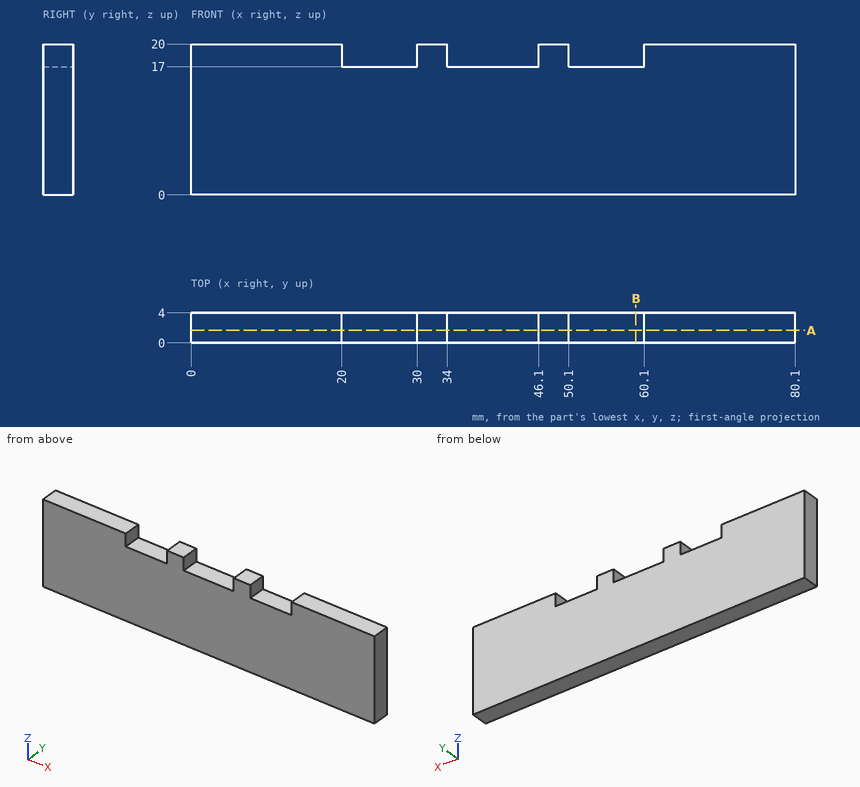
Study the drawing (mm; zero at the part's minimum x, y, z) and answer. Coordinates: 2 decimals unless noted, no trailing zeros. Order: outer loops, then holes, each group sorted by start corner. A loop starts at its lowest first (then second) coordinate and runs counter-clockwise, first axis right, second up. Notation, with made-up numbers: M 43,10 L 79,10 A36 cw 79,44 Z; hole C 82.25,51.25 d10. An arc over 180 degrees is marked long. Answer as a JSON object with one key per item and string values. Group by question number.
1. Section A-A on y = 1.65 is taken. Write down the section's boundary in (x, z), then the cut area to 3 significant figures.
2. Straight lines are drawn through the part: line 1 (X direction, y = 2.6, z = 17.5); line 2 (Z direction, x = 40.5, y = 1.4). For each, find the intervals that lie inside material, in ascending order.
3. A flat-ended cylindrical pin translates along its axis: P1, Ø1.2, axis at x = 24.5, y = 2.5, coming from the +Z side. Find the tip coordinate at first contact, or state that the pin passes through.
4. Section B-B on x = 59 is taken. Write down the section's boundary in (y, z).
Values follow:
{
 "1": {"outline": "M 0,0 L 80.1,0 L 80.1,20 L 60.1,20 L 60.1,17 L 50.1,17 L 50.1,20 L 46.1,20 L 46.1,17 L 34,17 L 34,20 L 30,20 L 30,17 L 20,17 L 20,20 L 0,20 Z", "area": "1,510 mm2"},
 "2": {"line 1": "0 to 20, 30 to 34, 46.1 to 50.1, 60.1 to 80.1", "line 2": "0 to 17"},
 "3": {"P1": "z = 17"},
 "4": {"outline": "M 0,0 L 4,0 L 4,17 L 0,17 Z"}
}
